For this review, take the finished solid that the model builds, in its own axes (mm). Face numbers are marked on the shaded views. Coordinates: 2 decimals unless noted, no trailing zeros. Loops run counter-clockwise (first coordinate to the right, second up) from the corner with the lowest first, then second, coordinate; pieces in that order, holes last. Notation, with made-up numbers: (1.5, 30.5) - (9.5, 30.5) arc R26 ccw to (9.5, 60.5) - close; hole circle Ø10 at (42, -15.75). An arc over 180 degrees is marked (long way). Answer as a JSON object with one key per item and string values. Group by question number.
Item 1: We need section B-B (y = 2.8). Give the boundary of the cut face in (x, z).
Item 2: We need section D-D (z = 0). Give the boundary of the cut face in (x, y).
Item 3: We need section C-C (x = 3). Give the boundary of the cut face in (y, z), then the cut area to 3 significant figures.
Item 4: Mouldability with a two-part tool opening along X and no side actions: class the marked faces 1, 2 and 3 as released by +X, released by -X, zero draft, split by the parting line, or undercut.
Item 5: We need section A-A (x = 0). State how many separate pieces and enclosed holes the cut face has, then the cut area to 3 significant figures.
Item 6: To check wall thickness, follow line 1 (Z direction, x = 0, y = 0.75); line 2 (Z direction, x = -3, y = 3.55); line 3 (X direction, y = 2.7, z = 0.5). State the ranges of each line that lie inside material, in increasing order.
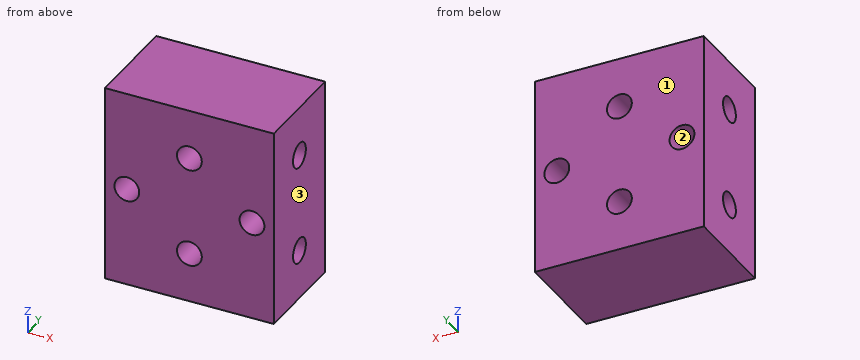
from build123d import *

# Parameters (mm, degrees)
SKETCH1_W                           = 8.1
SKETCH1_H                           = 9.525
BOSS_EXTRUDE1_DEPTH                 = 4.7625
F_0_80_TAPPED_HOLE1_D               = 1.19126
F_0_80_TAPPED_HOLE2_D               = 1.19126
F_3_64_0_04688_DIAMETER_HOLE1_D     = 1.190752
F_3_64_0_04688_DIAMETER_HOLE1_DEPTH = 12.954
F_3_64_0_04688_DIAMETER_HOLE1_TIP   = 0.357737992


with BuildPart() as part:
    # Sketch1 → Boss-Extrude1 (new body)
    with BuildSketch(Plane(origin=(0, 0, 0), x_dir=(1, 0, 0), z_dir=(0, 1, 0))):
        Rectangle(SKETCH1_W, SKETCH1_H)
    extrude(amount=BOSS_EXTRUDE1_DEPTH)

    # #0-80 Tapped Hole1 (through all)
    with Locations(Plane.ZY.offset(4.05)):
        with Locations((-2.38125, 2.38125), (2.38125, 2.38125)):
            Hole(F_0_80_TAPPED_HOLE1_D / 2)

    # #0-80 Tapped Hole2 (through all)
    with Locations(Plane.XZ):
        with Locations((-3, 0), (3, 0)):
            Hole(F_0_80_TAPPED_HOLE2_D / 2)

    # 3/64 (0.04688) Diameter Hole1
    with Locations(Plane(origin=(0, 4.7625, 0), x_dir=(-1, 0, 0), z_dir=(0, 1, 0))):
        with Locations((0, 2.38125), (0, -2.38125)):
            Hole(F_3_64_0_04688_DIAMETER_HOLE1_D / 2, depth=F_3_64_0_04688_DIAMETER_HOLE1_DEPTH)
            with Locations((0, 0, -(F_3_64_0_04688_DIAMETER_HOLE1_DEPTH + F_3_64_0_04688_DIAMETER_HOLE1_TIP / 2))):  # 118° drill point
                Cone(0, F_3_64_0_04688_DIAMETER_HOLE1_D / 2, F_3_64_0_04688_DIAMETER_HOLE1_TIP, mode=Mode.SUBTRACT)


solid = part.part
Check sheet entries:
{
 "1": {"outline": "(-4.05, -4.76) - (4.05, -4.76) - (4.05, -2.8) - (0.42, -2.8) arc R0.6 cw to (-0.42, -2.8) - (-4.05, -2.8) - close; (-4.05, -1.96) - (-0.42, -1.96) arc R0.6 cw to (0.42, -1.96) - (4.05, -1.96) - (4.05, 1.96) - (0.42, 1.96) arc R0.6 cw to (-0.42, 1.96) - (-4.05, 1.96) - close; (-4.05, 2.8) - (-0.42, 2.8) arc R0.6 cw to (0.42, 2.8) - (4.05, 2.8) - (4.05, 4.76) - (-4.05, 4.76) - close; hole circle Ø1.19 at (-3, 0); hole circle Ø1.19 at (3, 0)"},
 "2": {"outline": "(-4.05, 0) - (-3.6, 0) - (-3.6, 4.76) - (-4.05, 4.76) - close; (-2.4, 0) - (2.4, 0) - (2.4, 4.76) - (-2.4, 4.76) - close; (3.6, 0) - (4.05, 0) - (4.05, 4.76) - (3.6, 4.76) - close"},
 "3": {"outline": "(0, -4.76) - (4.76, -4.76) - (4.76, -0.6) - (0, -0.6) - close; (0, 0.6) - (4.76, 0.6) - (4.76, 4.76) - (0, 4.76) - close; hole circle Ø1.19 at (2.38, -2.38); hole circle Ø1.19 at (2.38, 2.38)", "area": "37.5 mm2"},
 "4": {"face 1": "zero draft", "face 2": "undercut", "face 3": "released by +X"},
 "5": {"separate pieces": "3", "enclosed holes": "0", "area": "34.0 mm2"},
 "6": {"line 1": "z = -4.76 to -2.98, -1.79 to 1.79, 2.98 to 4.76", "line 2": "z = -4.76 to -0.6, 0.6 to 4.76", "line 3": "x = -4.05 to -3.32, -2.68 to 2.68, 3.32 to 4.05"}
}
